```python
from build123d import *

# Parameters (mm, degrees)
SKETCH_1_W             = 2.54
SKETCH_1_H             = 2.54
EXTRUDE_1_DEPTH        = 2.54
CHAMFER_1_SIZE         = 0.4
SKETCH_2_W             = 0.65
SKETCH_2_H             = 0.65
EXTRUDE_2_DEPTH        = 5.8
EXTRUDE_START          = -2.54
SKETCH_2_2_W           = 0.65
SKETCH_2_2_H           = 0.65
EXTRUDE_3_DEPTH        = 2.5
CHAMFER_2_SIZE         = 0.6
CHAMFER_2_SIZE2        = 0.1
CHAMFER_2_PART_2_SIZE  = 0.6
CHAMFER_2_PART_2_SIZE2 = 0.1
CHAMFER_2_PART_3_SIZE  = 0.6
CHAMFER_2_PART_3_SIZE2 = 0.1
CHAMFER_2_PART_4_SIZE  = 0.6
CHAMFER_2_PART_4_SIZE2 = 0.1
CHAMFER_3_SIZE         = 0.1
CHAMFER_3_SIZE2        = 0.6


with BuildPart() as part:
    # Эскиз1 → Бобышка-Вытянуть1 (new body)
    with BuildSketch(Plane(origin=(0, 0, 0), x_dir=(1, 0, 0), z_dir=(0, 1, 0))):
        Rectangle(SKETCH_1_W, SKETCH_1_H)
    extrude(amount=EXTRUDE_1_DEPTH)

    # Фаска1
    chamfer_1_edges = [part.edges().sort_by_distance(p)[0] for p in [
        (-1.27, 1.27, -1.27),
        (1.27, 1.27, -1.27),
        (1.27, 1.27, 1.27),
        (-1.27, 1.27, 1.27),
    ]]
    chamfer(chamfer_1_edges, length=CHAMFER_1_SIZE)

    # Эскиз2 → Бобышка-Вытянуть2 (add)
    with BuildSketch(Plane(origin=(0, 2.54, 0), x_dir=(1, 0, 0), z_dir=(0, 1, 0))):
        Rectangle(SKETCH_2_W, SKETCH_2_H)
    extrude(amount=EXTRUDE_2_DEPTH)

    # Эскиз2<2> → Бобышка-Вытянуть3 (add)
    with BuildSketch(Plane(origin=(0, 2.54, 0), x_dir=(1, 0, 0), z_dir=(0, 1, 0)).offset(EXTRUDE_START)):
        Rectangle(SKETCH_2_2_W, SKETCH_2_2_H)
    extrude(amount=-EXTRUDE_3_DEPTH)

    # Фаска2
    chamfer_2_edges = [part.edges().sort_by_distance(p)[0] for p in [
        (-0.325, 8.34, 0),
    ]]
    chamfer_2_side = [part.faces().sort_by_distance(p)[0] for p in [
        (-0.325, 5.44, 0),
    ]]
    chamfer(chamfer_2_edges, length=CHAMFER_2_SIZE, length2=CHAMFER_2_SIZE2, reference=chamfer_2_side[0])

    # Фаска2 part 2
    chamfer_2_part_2_edges = [part.edges().sort_by_distance(p)[0] for p in [
        (0, 8.34, 0.325),
    ]]
    chamfer_2_part_2_side = [part.faces().sort_by_distance(p)[0] for p in [
        (0, 5.44, 0.325),
    ]]
    chamfer(chamfer_2_part_2_edges, length=CHAMFER_2_PART_2_SIZE, length2=CHAMFER_2_PART_2_SIZE2, reference=chamfer_2_part_2_side[0])

    # Фаска2 part 3
    chamfer_2_part_3_edges = [part.edges().sort_by_distance(p)[0] for p in [
        (0.325, 8.34, 0),
    ]]
    chamfer_2_part_3_side = [part.faces().sort_by_distance(p)[0] for p in [
        (0.325, 5.44, 0),
    ]]
    chamfer(chamfer_2_part_3_edges, length=CHAMFER_2_PART_3_SIZE, length2=CHAMFER_2_PART_3_SIZE2, reference=chamfer_2_part_3_side[0])

    # Фаска2 part 4
    chamfer_2_part_4_edges = [part.edges().sort_by_distance(p)[0] for p in [
        (0, 8.34, -0.325),
    ]]
    chamfer_2_part_4_side = [part.faces().sort_by_distance(p)[0] for p in [
        (0, 5.44, -0.325),
    ]]
    chamfer(chamfer_2_part_4_edges, length=CHAMFER_2_PART_4_SIZE, length2=CHAMFER_2_PART_4_SIZE2, reference=chamfer_2_part_4_side[0])

    # Фаска3
    chamfer_3_edges = [part.edges().sort_by_distance(p)[0] for p in [
        (-0.325, -2.5, 0),
        (0, -2.5, -0.325),
        (0.325, -2.5, 0),
        (0, -2.5, 0.325),
    ]]
    chamfer_3_side = [part.faces().sort_by_distance(p)[0] for p in [
        (0, -2.5, 0),
    ]]
    chamfer(chamfer_3_edges, length=CHAMFER_3_SIZE, length2=CHAMFER_3_SIZE2, reference=chamfer_3_side[0])


solid = part.part
```
Geometry: final body of the model. Coordinates: model frame, mm. A direction names the side the tool comes from. Round coordinates to 2 decimals unless told otherwise and drop trailing zeros. Loops run counter-clockwise (first coordinate to the right, second up) from the corner with the lowest first, then second, coordinate; pieces in that order, holes last. Notation, with made-up numbers: (79.5, 4.5) -> (132.5, 4.5) arc R11 ccw to (132.5, 16.5) -> close; hole circle Ø5 at (63.25, 40). An arc over 180 degrees is marked (long way). Use one line per item in the form item = value. Start each with the question number.
1) Section A-A on x = 0.1. Output: boundary loops of the cut face in (y, z) (3 decimals), then the cut area to 3 significant figures.
2) Access query for faces 1 (the flat face through (1.27, 1, 0)), 2 (the flat face through (1, 2.54, 0)). Directions: +Z, -Z, +X, -X, +Y, -Y. A direction counts if a zero-diameter tool reaches every point of the face in a straight line with its end or side. Return the directions, or none.
3) Section B-B on z = 0.1. Output: boundary loops of the cut face in (x, y) (3 decimals).
4) Line query: L1, parallel to Y at x = -1.1, z = -0.3; L2, parallel to X at y = 3, z = 0.25 (3 decimals). Output: solid intervals per line, ascending.
5) Section C-C on y = 1. Output: boundary loops of the cut face in (x, z), then the cut area to 3 significant figures.
6) First-contact query: P1, Ø0.5, axis at y = -1, z = 0, coming from the -X side (3 decimals); P2, Ø0.7, axis at x = 0, y = 5.5, coming from the +Z side (3 decimals); P3, Ø0.5, axis at y = 4, z = 0, coming from the +X side (3 decimals). Flat tips, straight axial feed; report the tip coordinate or a pass-through.
7) Section D-D on x = -0.65. Output: boundary loops of the cut face in (y, z).
Response:
q1.outline = (-2.5, -0.225) -> (-1.9, -0.325) -> (0, -0.325) -> (0, -1.27) -> (2.54, -1.27) -> (2.54, -0.325) -> (7.74, -0.325) -> (8.34, -0.225) -> (8.34, 0.225) -> (7.74, 0.325) -> (2.54, 0.325) -> (2.54, 1.27) -> (0, 1.27) -> (0, 0.325) -> (-1.9, 0.325) -> (-2.5, 0.225) -> close
q1.area = 11.7 mm^2
q2.face_1 = +Z, -Z, +X, +Y, -Y
q2.face_2 = +Y
q3.outline = (-1.27, 0) -> (-0.325, 0) -> (-0.325, -1.9) -> (-0.225, -2.5) -> (0.225, -2.5) -> (0.325, -1.9) -> (0.325, 0) -> (1.27, 0) -> (1.27, 2.54) -> (0.325, 2.54) -> (0.325, 7.74) -> (0.225, 8.34) -> (-0.225, 8.34) -> (-0.325, 7.74) -> (-0.325, 2.54) -> (-1.27, 2.54) -> close
q4.L1 = 0 to 2.54
q4.L2 = -0.325 to 0.325
q5.outline = (-1.27, -0.87) -> (-0.87, -1.27) -> (0.87, -1.27) -> (1.27, -0.87) -> (1.27, 0.87) -> (0.87, 1.27) -> (-0.87, 1.27) -> (-1.27, 0.87) -> close
q5.area = 6.13 mm^2
q6.P1 = -0.325
q6.P2 = 0.325
q6.P3 = 0.325
q7.outline = (0, -1.27) -> (2.54, -1.27) -> (2.54, 1.27) -> (0, 1.27) -> close
